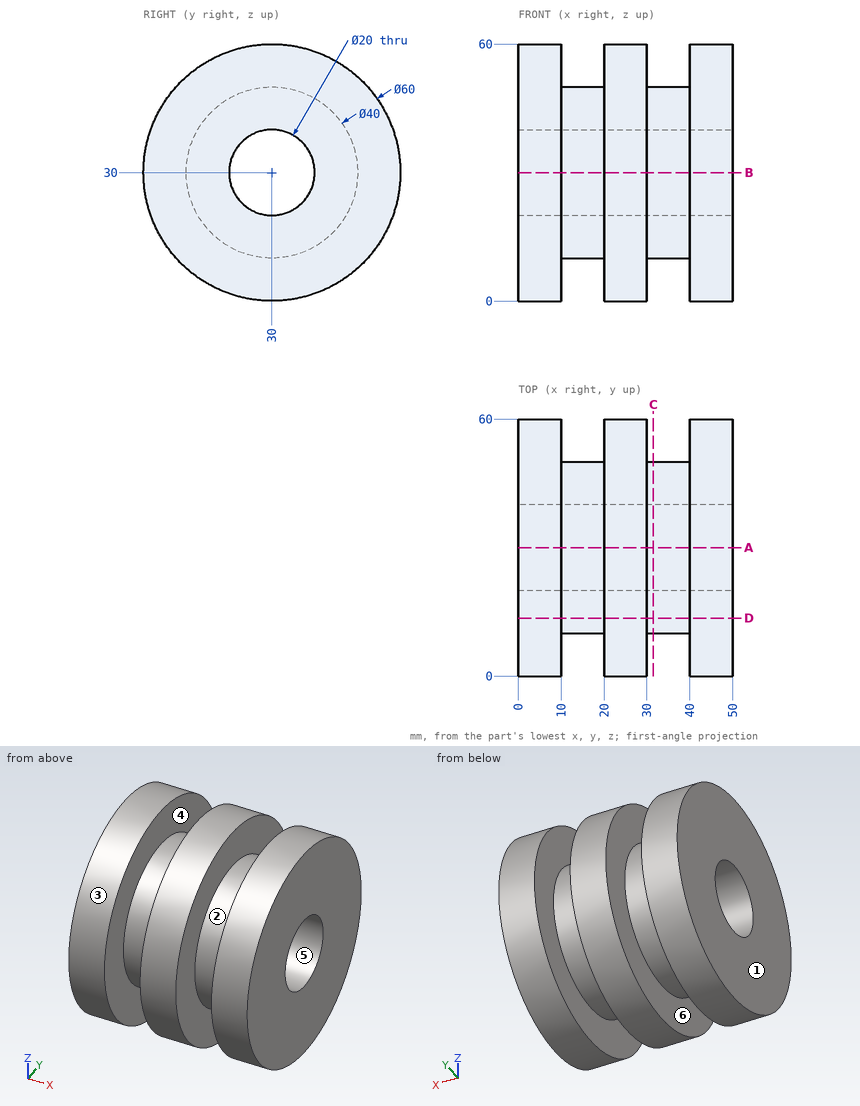
Answer from the drawing. Dimensions are ordinates in mm from the lowest x, y and z of the part. A direction names the side the tool comes from. Give positions to 0.01 mm unless a question says otherwise; leave off trailing zeros. Loops run counter-clockwise (first coordinate to the right, second up) from the corner with the lowest first, then second, coordinate; pieces in that order, holes last. Notation, with made-up numbers: (60.25, -26) -> (92.25, -26) arc R35 cw to (92.25, 7) -> close; hole circle Ø10 at (55, 21). An arc over 180 degrees is marked (long way). One line per question, with ' | ' between items. Start each with the question number.
1) For the marked faces 5 and 6, determine the directions among +Z, -Z, +X, -X, +Y, -Y from which every point of the face is accessible in a straight line to the end or side of a thin tool.
2) Section D-D, the plane y = 13.5 is taken. Determine the outline of the cut face in (x, z).
3) Section A-A, the plane y = 30 is taken. Determine the outline of the cut face in (x, z), then the cut area to 3 significant figures.
4) Determine the mould class of the marked faces 1, 2, 3 and 4 for opening direction X: +X half, -X half, draft (parallel to the pull), parting line (faces both ways), or undercut.
5) Each of these flat-tipped pins is pushed along its axis until it touches: pin 1 (1 mm diameter, centred on x = 41.5, z = 27, fed in from -Y); pin 2 (18 mm diameter, centred on y = 29.5, z = 19.5, fed in from -X); pin 3 (12 mm diameter, centred on x = 20.5, y = 31, fed in from -Z); pin 4 (6 mm diameter, centred on x = 11.5, z = 51.5, fed in from +Y). Where does it stop, or does it pass through?
6) Section C-C, the plane x = 31.5 is taken. Determine the outline of the cut face in (y, z).
7) Straight lines are drawn through the part: L1, parallel to X at y = 16.5, z = 51; L2, parallel to Z at x = 16.5, y = 30; L3, parallel to Z at x = 26, y = 30. For each, find the intervals that lie inside material, in ascending order.
Resolved:
1) face 5: +X, -X | face 6: none
2) outline: (0, 4.95) -> (10, 4.95) -> (10, 18.7) -> (20, 18.7) -> (20, 4.95) -> (30, 4.95) -> (30, 18.7) -> (40, 18.7) -> (40, 4.95) -> (50, 4.95) -> (50, 55.05) -> (40, 55.05) -> (40, 41.3) -> (30, 41.3) -> (30, 55.05) -> (20, 55.05) -> (20, 41.3) -> (10, 41.3) -> (10, 55.05) -> (0, 55.05) -> close
3) outline: (0, 0) -> (10, 0) -> (10, 10) -> (20, 10) -> (20, 0) -> (30, 0) -> (30, 10) -> (40, 10) -> (40, 0) -> (50, 0) -> (50, 20) -> (0, 20) -> close; (0, 40) -> (50, 40) -> (50, 60) -> (40, 60) -> (40, 50) -> (30, 50) -> (30, 60) -> (20, 60) -> (20, 50) -> (10, 50) -> (10, 60) -> (0, 60) -> close | area: 1,600 mm2
4) face 1: -X half | face 2: undercut | face 3: draft | face 4: undercut
5) pin 1: y = 0.1 | pin 2: x = 0 | pin 3: z = 0 | pin 4: y = 53.3
6) outline: circle Ø40 at (30, 30); hole circle Ø20 at (30, 30)
7) L1: 0 to 10, 20 to 30, 40 to 50 | L2: 10 to 20, 40 to 50 | L3: 0 to 20, 40 to 60
